from build123d import *

# Parameters (mm, degrees)
F_8_CLEARANCE_HOLE1_D = 4.4958


with BuildPart() as part:
    # Sketch1 → Revolve1 (revolve)
    with BuildSketch(Plane(origin=(0, 0, 0), x_dir=(0, 0, -1), z_dir=(1, 0, 0))):
        Polygon((0, -7), (0, 7), (-13.112500064, 7), (-13.112500064, 6), (-7.9375, 6), (-7.9375, -6), (-13.112500064, -6), (-13.112500064, -7), align=None)
    revolve(axis=Axis((0, -7, 0), (0, 1, 0)))

    # #8 Clearance Hole1 (through all)
    with Locations(Plane(origin=(0, 7, 0), x_dir=(1, 0, 0), z_dir=(0, 1, 0))):
        with Locations((0, 0)):
            Hole(F_8_CLEARANCE_HOLE1_D / 2)


solid = part.part
Build history of the part. All positions in model axes, mm. A direction names the side the tool comes from. Give positions to 0.01 mm unless a question says otherwise; leave off trailing zeros. Order: outer loops, then holes, each group sorted by start corner. A loop starts at its lowest first (then second) coordinate and runs counter-clockwise, first axis right, second up. Notation, with made-up numbers: M 13.5,65.25 L 30.5,65.25 A25 ccw 30.5,97.25 Z; hole C -33.75,65 d6. An arc over 180 degrees is marked long. Put each result on its own line as item: value.
Item 1: Drop flat-ended pins along their axis: pin 1 Ø8 at (y, z) = (-0.5, 0) entering from +X; pin 2 Ø1.5 at (x, y) = (-5.5, -5.5) entering from +Z; pin 3 Ø5 at (y, z) = (2.5, -2.5) entering from -X. Give the stop position or say it passes through.
Results are:
pin 1: x = 7.94
pin 2: z = 12.15
pin 3: x = -7.94
Item 2: Cut at D-D on x = 8.75. Write the cut outline in (y, z).
Results are:
outline: M -7,-9.77 L -6,-9.77 L -6,9.77 L -7,9.77 Z; M 6,-9.77 L 7,-9.77 L 7,9.77 L 6,9.77 Z
Item 3: Wall check: probe 1 along Y at (x, z) = (3.75, 11); probe 2 along X at (y, z) = (4.25, 1.25); probe 3 along Z at (x, y) = (3.75, 2.75). Give the ranges that are in metal, low to high.
Results are:
probe 1: -7 to -6, 6 to 7
probe 2: -7.84 to -1.87, 1.87 to 7.84
probe 3: -7 to 7
Item 4: Which spindle directions (+Z, -Z, +X, -X, +Y, -Y) get a long thin tool onto all of the face, cutting with end or side? Do faces 1 (the face through (-6, 6, 6)), 2 (the face through (-3, -7, 0)). Say none if no direction does.
Results are:
face 1: none
face 2: +Z, -Z, +X, -X, -Y
Item 5: Cut at A-A on x = 0. Write the cut outline in (y, z).
Results are:
outline: M -7,-13.11 L -6,-13.11 L -6,-7.94 L 6,-7.94 L 6,-13.11 L 7,-13.11 L 7,-2.25 L -7,-2.25 Z; M -7,2.25 L 7,2.25 L 7,13.11 L 6,13.11 L 6,7.94 L -6,7.94 L -6,13.11 L -7,13.11 Z
Item 6: Pull direction X, two halves, no side cores. Call faces 3 (the face through (-2.076, -0.098, 0.861)), 4 (the face through (-3, 7, 0)), 5 (the face through (3.939, 6.493, 12.507)): +X half, -X half, draft (parallel to the pull), parting line (faces both ways), or undercut.
Results are:
face 3: undercut
face 4: draft
face 5: parting line
Item 7: Cut at B-B on z = 0. Write the cut outline in (x, y).
Results are:
outline: M -13.11,-7 L -2.25,-7 L -2.25,7 L -13.11,7 L -13.11,6 L -7.94,6 L -7.94,-6 L -13.11,-6 Z; M 2.25,-7 L 13.11,-7 L 13.11,-6 L 7.94,-6 L 7.94,6 L 13.11,6 L 13.11,7 L 2.25,7 Z
Item 8: Cut at C-C on z = 11.25. Write the cut outline in (x, y), then the cut area to 3 significant figures.
Results are:
outline: M -6.74,-7 L 6.74,-7 L 6.74,-6 L -6.74,-6 Z; M -6.74,6 L 6.74,6 L 6.74,7 L -6.74,7 Z
area: 26.9 mm2
